from build123d import *

# Parameters (mm, degrees)
BOSS_EXTRUDE1_DEPTH = 12.3
CUT_EXTRUDE1_DEPTH  = 13.3


with BuildPart() as part:
    # Sketch1 → Boss-Extrude1 (new body)
    with BuildSketch(Plane(origin=(0, 0, 0), x_dir=(1, 0, 0), z_dir=(0, 1, 0))):
        with BuildLine():
            ThreePointArc((0, 0), (27.937327101, 23.623695395), (55.874654202, 0))
            ThreePointArc((55.874654202, 0), (27.937327101, -7.03951799), (0, 0))
        make_face()
    extrude(amount=BOSS_EXTRUDE1_DEPTH)

    # Sketch2 → Cut-Extrude1 (cut, through all)
    with BuildSketch(Plane(origin=(0, 12.3, 0), x_dir=(1, 0, 0), z_dir=(0, 1, 0))):
        with BuildLine():
            ThreePointArc((6.512863529, 0), (9.77491486, 5.638211193), (14.304676712, 10.319200608))
            ThreePointArc((14.304676712, 10.319200608), (16.969047295, 14.945891186), (22.305064172, 14.766837577))
            ThreePointArc((22.305064172, 14.766837577), (26.593603486, 17.95377667), (31.656828978, 16.247348283))
            ThreePointArc((31.656828978, 16.247348283), (36.195985479, 17.887121813), (39.87791775, 14.766837577))
            ThreePointArc((39.87791775, 14.766837577), (44.568649172, 14.965090252), (47.03719079, 10.971524469))
            ThreePointArc((47.03719079, 10.971524469), (52.083128874, 6.059747982), (55.670118393, 0))
            ThreePointArc((55.670118393, 0), (31.091490961, -3.658407288), (6.512863529, 0))
        make_face()
    extrude(amount=-CUT_EXTRUDE1_DEPTH, mode=Mode.SUBTRACT)


solid = part.part
Work out the finished part from the listing and answer in its coordinate system (mm). A direction names the side the tool comes from. Give positions to 0.01 mm unless a question says otherwise; leave off trailing zeros. Order: outer loops, then holes, each group sorted by start corner. A loop starts at its lowest first (then second) coordinate and runs counter-clockwise, first axis right, second up. Notation, with made-up numbers: (78, -19) - (124, -19) arc R27 cw to (124, 15) - close; hole circle Ø10 at (51.5, 50.25). An arc over 180 degrees is marked (long way). Answer as CSV lines item,"result". Start each with the question number.
Q1. For faces 1 (the face through (31.441, 6.236, 3.658)), 2 (the face through (22, 12.3, -16)), determine the directions among +Z, -Z, +X, -X, +Y, -Y from which every point of the face is accessible in a straight line to the end or side of a thin tool.
Q2. Find the intervals of material crossed by L1, parallel to X at y = 11.5, z = -15; L2, parallel to Z at x = 49.5, y = 1.75; L3, parallel to Z at x = 29.5, y = 1.5, in increasing order. Write a range as [from, to].
Q3. The part is cut by section B-B (x = 16.5). Write down the section's boundary in (y, z).
Q4. The part is cut by section A-A (z = -13). Write down the section's boundary in (x, y), then the cut area to 3 significant figures.
Q5. The mould has two halves that part along Z. Classify faces 3 (the face through (22, 0, -16)), 4 (the face through (28.34, 6.06, 7.04)), 5 (the face through (9.72, 6.236, -5.565)), 6 (the face through (44.5, 6.2, -15)): +Z half, -Z half, draft (parallel to the pull), parting line (faces both ways), or undercut.
Q6. The part is cut by section C-C (y = 7.25). Write down the section's boundary in (x, z).
Q7. Given pin 1 Ø1 at (x, y) = (38.5, 4.5) entering from +Z; pin 2 Ø4 at (y, z) = (4, -10.5) entering from -X; pin 3 Ø6 at (y, z) = (6.5, -12) entering from +X, each flat-ended and moving along its own axis, determine where each tip first touches the part or whether it passes through.
Q8. The part is cut by section D-D (z = -19). Write down the section's boundary in (x, y), then the cut area to 3 significant figures.
Check result:
1,face 1,"+Y, -Y"
1,face 2,"+Z, -Z, +X, -X, +Y"
2,L1,"x = [7.58, 17.07], [21.91, 22.42], [39.79, 40.28], [44.5, 48.29]"
2,L2,"z = [-13.67, -8.9], [1.63, 2.95]"
2,L3,"z = [-23.58, -17.66], [3.64, 7.02]"
3,outline,"(0, -21.21) - (12.3, -21.21) - (12.3, -14.65) - (0, -14.65) - close; (0, 2.39) - (12.3, 2.39) - (12.3, 5.92) - (0, 5.92) - close"
4,outline,"(5.82, 0) - (14.99, 0) - (14.99, 12.3) - (5.82, 12.3) - close; (46.52, 0) - (50.05, 0) - (50.05, 12.3) - (46.52, 12.3) - close"
4,area,"156 mm²"
5,face 3,"draft"
5,face 4,"+Z half"
5,face 5,"undercut"
5,face 6,"undercut"
6,outline,"(0, 0) arc R28.33 ccw to (55.87, 0) arc R58.96 ccw to start; hole (6.51, 0) arc R26.71 ccw to (14.3, -10.32) arc R5.18 ccw to (22.31, -14.77) arc R5.76 ccw to (31.66, -16.25) arc R4.82 ccw to (39.88, -14.77) arc R4.65 ccw to (47.04, -10.97) arc R26.71 ccw to (55.67, 0) arc R84.39 ccw to start"
7,pin 1,"stops at z = 6.17"
7,pin 2,"stops at x = 2.87"
7,pin 3,"stops at x = 52.73"
8,outline,"(12.43, 0) - (43.45, 0) - (43.45, 12.3) - (12.43, 12.3) - close"
8,area,"382 mm²"
